Geometry check sheet. Reference: drawing and pictorial views, mm from the part's lowest x, y, z. A direction names the side the tool comes from. Give positions to 0.01 mm unless a question says otherwise; leave off trailing zeros. Write each loop counter-clockwise with the first axis right and the second up, starting at its lowest first coordinate (ties: lowest second). Pieces come first, ordered by that corner, then holes. Notation, with made-up numbers: (-30, -12) -> (9, -12) arc R30 ccw to (9, 17) -> close; hole circle Ø11 at (60.5, 63). An arc over 180 degrees is marked (long way). Return JSON: item names as keys, results as strings.
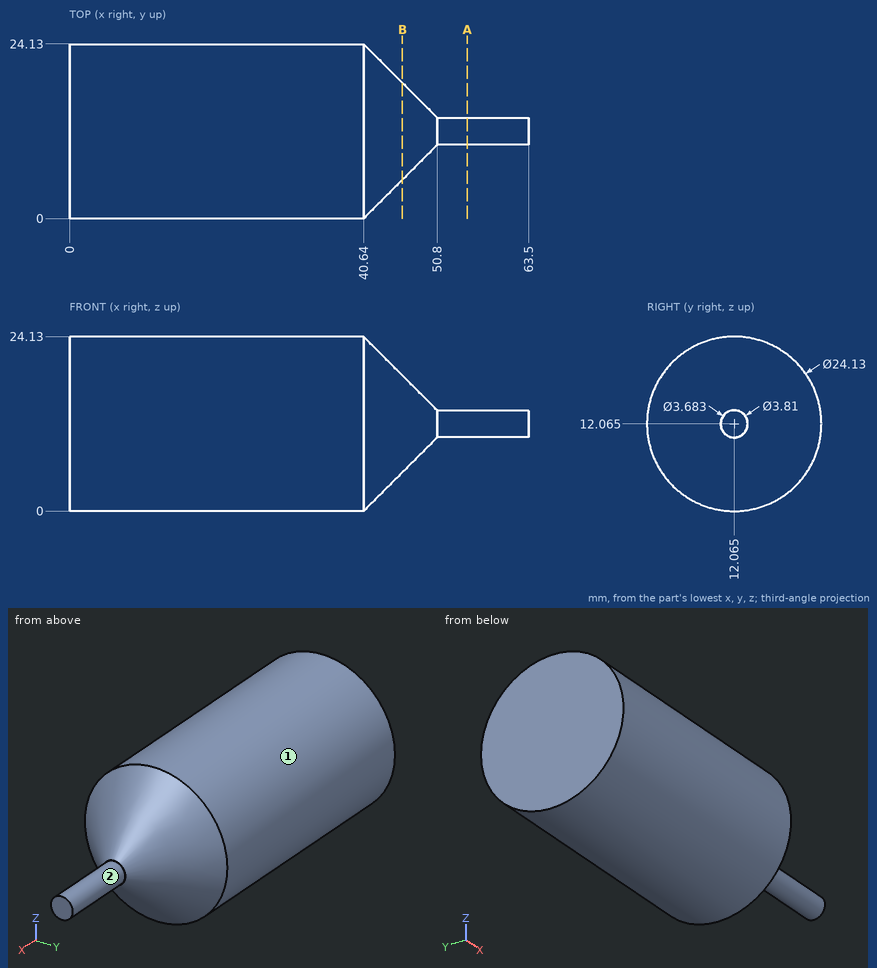
(1) Depth check by flat-ended pin: pin 1 Ø10 at (x, y) = (50, 18.5) entering from +Z; pin 2 Ø5 at (x, z) = (11.5, 20.5) entering from +Y. Enter the tip coordinate at first touch or a pass-through.
Reply:
{"pin 1": "z = 17.9", "pin 2": "y = 22.57"}
(2) Thickness scan on L1, parallel to Z at x = 15.5, y = 11.75; L2, parallel to X at y = 13.75, z = 18; L3, parallel to X at y = 17, z = 20.5. Record the ranges inside material, lowest first.
Reply:
{"L1": "0 to 24.13", "L2": "0 to 46.54", "L3": "0 to 42.93"}
(3) Cross-section at B-B on x = 46. Enter the section's corners in (y, z) (3 decimals), then the cut area to 3 significant figures.
Reply:
{"outline": "circle Ø13.41 at (12.065, 12.065)", "area": "141 mm^2"}
(4) Set-up check for the marked faces 1 and 2: record each of +Z, -Z, +X, -X, +Y, -Y from which the full face is reachable in a straight line by a thin tool's end or side.
Reply:
{"face 1": "+X, -X", "face 2": "+X"}
(5) Cross-section at A-A on x = 55. Enter the section's corners in (y, z) (1 decimal), then the cut area to 3 significant figures.
Reply:
{"outline": "circle Ø3.7 at (12.1, 12.1)", "area": "10.7 mm^2"}
